Verification items for this drawing (mm, ordinates from the low corner). Coordinates: 2 decimals unless noted, no trailing zeros. Order: outer loops, then holes, each group sorted by start corner. A loop starts at its lowest first (then second) coordinate and runs counter-clockwise, first axis right, second up. Notation, with made-up numbers: M 84.5,-5 L 135.5,-5 A29 cw 135.5,32 Z; hole C 56.5,45 d6. An arc over 180 degrees is marked long. Answer as a JSON object with one key per item and string values. Group by question number.
(1) Mould release check, pull along Y, two halves, no side actions. Record for the marked faces 1, 2, 3 and 4: released by +Y, released by -Y, zero draft, split by the parting line, or undercut.
(2) Cross-section at A-A (y = 2.54). Enter the section's corners in (x, z).
(3) Cross-section at B-B (z = 0.4). Count the separate pieces of the cut face and the enclosed holes in it.
(4) Material ranges on line 1 (Y direction, x = 2.54, z = 1.15); line 2 (Y direction, x = 2, z = 1.15); line 3 (Z direction, x = 2.5, y = 11), recorded low to high.
(5) Cross-section at C-C (x = 2.54). Enter the section's corners in (y, z).
(6) Gauge pin test, flat ends, axial feed: pin 1 Ø0.7 at (y, z) = (10, 2.5) entering from +X (1 decimal); pin 2 Ø1.2 at (x, z) = (9, 2.5) entering from -Y (1 decimal). Record the tip position at first contact, or that the pin passes through.
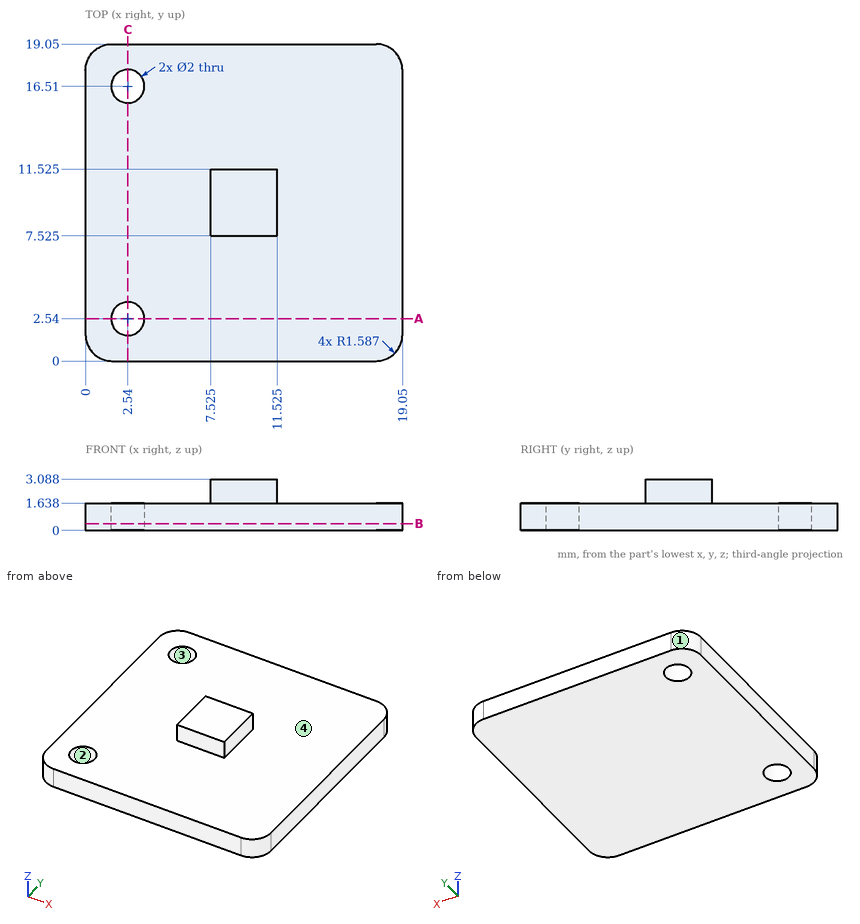
Taken from the geometry:
{
 "1": {"face 1": "released by +Y", "face 2": "undercut", "face 3": "undercut", "face 4": "zero draft"},
 "2": {"outline": "M 0,0 L 1.54,0 L 1.54,1.64 L 0,1.64 Z; M 3.54,0 L 19.05,0 L 19.05,1.64 L 3.54,1.64 Z"},
 "3": {"separate pieces": "1", "enclosed holes": "2"},
 "4": {"line 1": "y = 0 to 1.54, 3.54 to 15.51, 17.51 to 19.05", "line 2": "y = 0 to 1.7, 3.38 to 15.67, 17.35 to 19.05", "line 3": "z = 0 to 1.64"},
 "5": {"outline": "M 0,0 L 1.54,0 L 1.54,1.64 L 0,1.64 Z; M 3.54,0 L 15.51,0 L 15.51,1.64 L 3.54,1.64 Z; M 17.51,0 L 19.05,0 L 19.05,1.64 L 17.51,1.64 Z"},
 "6": {"pin 1": "stops at x = 11.5", "pin 2": "stops at y = 7.5"}
}
